```python
from build123d import *

# Parameters (mm, degrees)
ENL_V_MAT_EXTRU_1_REACH = 37.548


with BuildPart() as part:
    # Esquisse1 → Révolution1 (revolve)
    with BuildSketch(Plane.XY, mode=Mode.PRIVATE) as r_volution1_sk:
        Polygon((-1.5, 0), (-1.5, 33.7), (-2.925, 33.7), (-2.925, 3.3), (-4, 3.3), (-4, 3), (-8, 3), (-8, 0), align=None)
    revolve(r_volution1_sk.sketch.rotate(Axis((0, -3.664645975, 0), (0, 1, 0)), 270), axis=Axis((0, -3.664645975, 0), (0, 1, 0)))

    # Esquisse2 → Enlèv. mat.-Extru.1 (cut, up to next)
    with BuildSketch(Plane.XZ, mode=Mode.PRIVATE) as enl_v_mat_extru_1_sk1:
        with BuildLine():
            ThreePointArc((8, 0), (7.483314774, 2.828427125), (6, 5.291502622))
            Line((6, 5.291502622), (6, -5.291502622))
            ThreePointArc((6, -5.291502622), (7.483314774, -2.828427125), (8, 0))
        make_face()
    enl_v_mat_extru_1_tool1 = extrude(enl_v_mat_extru_1_sk1.sketch, amount=-ENL_V_MAT_EXTRU_1_REACH, mode=Mode.PRIVATE) & part.part
    # Esquisse2 → Enlèv. mat.-Extru.1 (cut, up to next)
    with BuildSketch(Plane.XZ, mode=Mode.PRIVATE) as enl_v_mat_extru_1_sk2:
        with BuildLine():
            Line((-6, -5.291502622), (-6, 5.291502622))
            ThreePointArc((-6, 5.291502622), (-8, 0), (-6, -5.291502622))
        make_face()
    enl_v_mat_extru_1_tool2 = extrude(enl_v_mat_extru_1_sk2.sketch, amount=-ENL_V_MAT_EXTRU_1_REACH, mode=Mode.PRIVATE) & part.part
    add(enl_v_mat_extru_1_tool1.solids().sort_by_distance((6.809243, 0, 0))[0], mode=Mode.SUBTRACT)
    add(enl_v_mat_extru_1_tool2.solids().sort_by_distance((-6.809243, 0, 0))[0], mode=Mode.SUBTRACT)


solid = part.part
```
The listing builds one solid part. Answer for the finished solid, in the listing's coordinates (mm). A direction names the side the tool comes from. Give positions to 0.01 mm unless a question says otherwise; leave off trailing zeros. Write each loop counter-clockwise with the first axis right and the second up, starting at its lowest first coordinate (ties: lowest second). Pieces come first, ordered by that corner, then holes. Notation, with made-up numbers: (24, 70.25) - (54, 70.25) arc R20 cw to (54, 108.25) - close; hole circle Ø11 at (21, -24.5). An arc over 180 degrees is marked (long way). Use one line per item in the form item = value. Start each with the question number.
1) A tool of negligible diameter and unlimited length cuts with its end or side. For faces 5 (the face through (1, 3.3, -3)), 6 (the face through (-6, 1, 0)), from which of +Z, -Z, +X, -X, +Y, -Y can it reach the whole face along a straight path? Write none if from no direction.
2) Find section D-D on x = -3.25. Determine the outline of the cut face in (y, z).
3) Find section A-A on x = 0. Determine the outline of the cut face in (y, z) (3 decimals).
4) The mould has two halves that part along Z. Classify faces 1 (the face through (0, 0, -2)), 2 (the face through (-0.45, 17.09, -1.43)), 3 (the face through (2.595, 18.287, -1.35)), 4 (the face through (0, 1, -8)): pulls with the +Z half, pulls with the -Z half, needs draft (parallel to the pull), parting line crosses it, or undercut.
5) Consider line 1 along X through (y, z) = (24, 0) (3 decimals); line 2 along Y through (x, z) = (4, 0.5); line 3 along Y through (x, z) = (-3.5, 1.75). Determine where each line is inside the solid, lowest interval first. Write a range as from..to.
6) Find section C-C on y = 26.5. Determine the outline of the cut face in (x, z) (3 decimals).
7) Find section B-B on z = 0. Determine the outline of the cut face in (x, y) (3 decimals).
8) Flat-ended cylindrical pins translate along their axes: pin 1 Ø1.5 at (x, y) = (-2.5, 24) entering from -Z; pin 2 Ø3 at (x, y) = (-4, 10) entering from +Z; pin 3 Ø4 at (x, y) = (-3, 25) entering from +Z. Find the tip coordinate at first contact, or state that the pin passes through.
Geometry results:
q1.face_5 = +Y
q1.face_6 = +Z, -Z, -X, +Y, -Y
q2.outline = (0, -7.31) - (3, -7.31) - (3, -2.33) - (3.3, -2.33) - (3.3, 2.33) - (3, 2.33) - (3, 7.31) - (0, 7.31) - close
q3.outline = (0, -8) - (3, -8) - (3, -4) - (3.3, -4) - (3.3, -2.925) - (33.7, -2.925) - (33.7, -1.5) - (0, -1.5) - close; (0, 1.5) - (33.7, 1.5) - (33.7, 2.925) - (3.3, 2.925) - (3.3, 4) - (3, 4) - (3, 8) - (0, 8) - close
q4.face_1 = needs draft
q4.face_2 = undercut
q4.face_3 = parting line crosses it
q4.face_4 = pulls with the -Z half
q5.line_1 = -2.925..-1.5, 1.5..2.925
q5.line_2 = 0..3
q5.line_3 = 0..3.3
q6.outline = circle Ø5.85 at (0, 0); hole circle Ø3 at (0, 0)
q7.outline = (-6, 0) - (-1.5, 0) - (-1.5, 33.7) - (-2.925, 33.7) - (-2.925, 3.3) - (-4, 3.3) - (-4, 3) - (-6, 3) - close; (1.5, 0) - (6, 0) - (6, 3) - (4, 3) - (4, 3.3) - (2.925, 3.3) - (2.925, 33.7) - (1.5, 33.7) - close
q8.pin_1 = -2.34
q8.pin_2 = 1.52
q8.pin_3 = 2.75
